```python
from build123d import *

# Parameters (mm, degrees)
F0_R      = 21.25
F1_DEPTH  = 66.03
F2_R      = 2
F3_R      = 21
F3_R_2    = 19.25
F4_DEPTH  = 5
F5_R      = 20.95
F6_DEPTH  = 35.9
F7_R      = 21
F7_R_2    = 20.95
F8_DEPTH  = 5
F9_R      = 10
F10_DEPTH = 2
F11_R     = 5
F12_DEPTH = 3
F13_R     = 4
F14_DEPTH = 19
F16_DEPTH = 12
F18_D     = 3.3
F18_DEPTH = 8.1
F18_TIP   = 0.9914200214
F19_R     = 1


with BuildPart() as f1:
    # F0 (on Front) → F1 (new body)
    with BuildSketch(Plane.XZ):
        Circle(F0_R)
    extrude(amount=F1_DEPTH)

    # F2
    f2_edges = [f1.edges().sort_by_distance(p)[0] for p in [
        (-21.25, -66.03, 0),
    ]]
    fillet(f2_edges, radius=F2_R)

    # F3 (on face) → F4 (join)
    with BuildSketch(Plane.XZ.offset(66.03)):
        Circle(F3_R)
        Circle(F3_R_2, mode=Mode.SUBTRACT)
        Circle(F3_R_2)
    extrude(amount=F4_DEPTH)

    # F5 (on face) → F6 (join)
    with BuildSketch(Plane.XZ.offset(71.03)):
        Circle(F5_R)
    extrude(amount=F6_DEPTH)

    # F7 (on face) → F8 (join)
    with BuildSketch(Plane.XZ.offset(106.93)):
        Circle(F7_R)
        Circle(F7_R_2, mode=Mode.SUBTRACT)
        Circle(F7_R_2)
    extrude(amount=F8_DEPTH)

    # F9 (on face) → F10 (join)
    with BuildSketch(Plane.XZ.offset(111.93)):
        with BuildLine():
            Line((11.5, -4.8989794856), (11.5, 4.8989794856))
            ThreePointArc((11.5, 4.8989794856), (0, 12.5), (-11.5, 4.8989794856))
            Line((-11.5, 4.8989794856), (-11.5, -4.8989794856))
            ThreePointArc((-11.5, -4.8989794856), (0, -12.5), (11.5, -4.8989794856))
        make_face()
        Circle(F9_R, mode=Mode.SUBTRACT)
    extrude(amount=F10_DEPTH)

    # F11 (on face) → F12 (join)
    with BuildSketch(Plane.XZ.offset(111.93)):
        Circle(F11_R)
    extrude(amount=F12_DEPTH)

    # F13 (on face) → F14 (join)
    with BuildSketch(Plane.XZ.offset(114.93)):
        Circle(F13_R)
    extrude(amount=F14_DEPTH)

    # F15 (on face) → F16 (cut)
    with BuildSketch(Plane.XZ.offset(133.93)):
        with BuildLine():
            Line((-2.6457513111, 3), (2.6457513111, 3))
            ThreePointArc((2.6457513111, 3), (0, 4), (-2.6457513111, 3))
        make_face()
    extrude(amount=-F16_DEPTH, mode=Mode.SUBTRACT)

    # F18
    with Locations(Plane.XZ.offset(111.93)):
        with Locations((-12.3743686708, 12.3743686708), (12.3743686708, 12.3743686708), (12.3743686708, -12.3743686708), (-12.3743686708, -12.3743686708)):
            Hole(F18_D / 2, depth=F18_DEPTH)
            with Locations((0, 0, -(F18_DEPTH + F18_TIP / 2))):  # 118° drill point
                Cone(0, F18_D / 2, F18_TIP, mode=Mode.SUBTRACT)

    # F19
    f19_edges = [f1.edges().sort_by_distance(p)[0] for p in [
        (-21, -66.03, 0),
        (-21, -111.93, 0),
    ]]
    fillet(f19_edges, radius=F19_R)


solid = f1.part
```
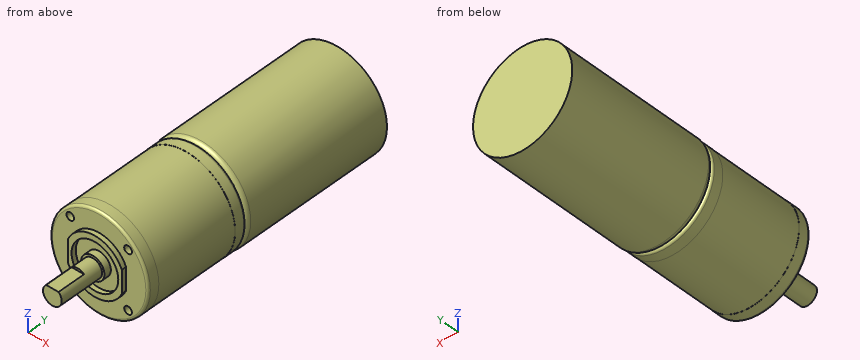
The listing builds one solid part. Answer for the finished solid, in the listing's coordinates (mm). Give positions to 0.01 mm unless a question says otherwise; leave off trailing zeros. Loops run counter-clockwise (first coordinate to the right, second up) from the corner with the lowest first, then second, coordinate; pieces in that order, holes last. Notation, with made-up numbers: M 53.25,-34 L 104.25,-34 A12 ccw 104.25,-15 Z; hole C 70,41 d1. An arc over 180 degrees is marked long. One line per item, written item: value.
1. Find the intervals of material crossed by probe 1 along Y at (x, z) = (10, 6); probe 2 along Y at (x, z) = (6, -17.5); probe 3 along X at (y, z) = (-112, 11.5), in increasing order.
Found:
probe 1: -113.93 to 0
probe 2: -111.93 to 0
probe 3: -4.9 to 4.9
2. Section A-A on y = -20 is taken. Determine the outline of the cut face in (x, z), plus the area to 3 significant figures.
Found:
outline: C 0,0 d42.5
area: 1,420 mm^2
3. Section B-B on y = -87.5 is taken. Determine the outline of the cut face in (x, z).
Found:
outline: C 0,0 d41.9
4. Each of these flat-tipped pins is pushed along its axis until it touches: P1, Ø3, axis at x = 12.37, z = 12.37, coming from the +Y side; P2, Ø4, axis at x = -7.5, y = -104.5, coming from the -Z side; P3, Ø10, axis at x = 12, z = 5.5, coming from the -Y side; P4, Ø10, axis at x = -16, y = -77, coming from the -Z side. Where does it stop, or does it pass through?
Found:
P1: y = 0
P2: z = -20.22
P3: y = -113.93
P4: z = -17.83
